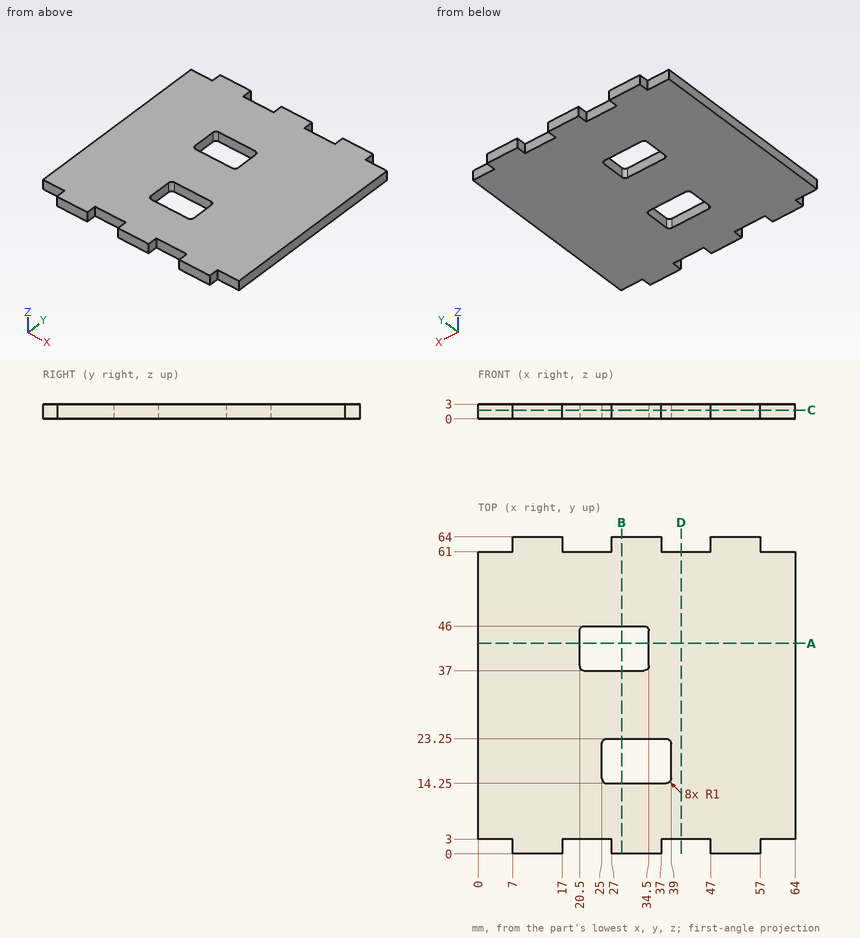
For this review, use the dimensioned drawing (mm, ordinates from the lowest corner) and the shaded views. Give positions to 0.01 mm unless a question says otherwise; leave off trailing zeros. Write each loop counter-clockwise with the first axis right and the second up, starting at its lowest first coordinate (ties: lowest second). Pieces come first, ordered by that corner, then holes. Notation, with made-up numbers: M -15,-13.75 L 21,-13.75 A18 ccw 21,-4.75 Z; hole C 2.25,44 d8. An arc over 180 degrees is marked long. Answer as a JSON object with one key per item and string values. Group by question number.
1) Clearance check with flat-ended pins moving along their axes: pin 1 Ø0.9 at (y, z) = (41, 1) entering from -X; pin 2 Ø1.5 at (y, z) = (63, 1) entering from +X; pin 3 Ø0.9 at (x, z) = (5, 2) entering from -Y. State where each tip first meets the part, or that it passes through.
2) We need section C-C (z = 1.75). Count the separate pieces of the cut face and the enclosed holes in it, and give its area (3 significant figures).
3) We need section A-A (y = 42.5). Give the boundary of the cut face in (x, z), and give its area (3 significant figures).
4) We need section D-D (x = 41). Give the boundary of the cut face in (y, z).
5) We need section B-B (x = 29). Give the boundary of the cut face in (y, z), and give its area (3 significant figures).
6) For line 1 along X through (y, z) = (42, 1.8); line 2 along Y through (x, z) = (24.5, 0.7); line 3 along Y through (x, z) = (25.5, 2.65), list the stretches that pass through material, from the lowest coordinate up.
Answer key:
{
 "1": {"pin 1": "stops at x = 0", "pin 2": "stops at x = 57", "pin 3": "stops at y = 3"},
 "2": {"separate pieces": "1", "enclosed holes": "2", "area": "3,640 mm²"},
 "3": {"outline": "M 0,0 L 20.5,0 L 20.5,3 L 0,3 Z; M 34.5,0 L 64,0 L 64,3 L 34.5,3 Z", "area": "150 mm²"},
 "4": {"outline": "M 3,0 L 61,0 L 61,3 L 3,3 Z"},
 "5": {"outline": "M 0,0 L 14.25,0 L 14.25,3 L 0,3 Z; M 23.25,0 L 37,0 L 37,3 L 23.25,3 Z; M 46,0 L 64,0 L 64,3 L 46,3 Z", "area": "138 mm²"},
 "6": {"line 1": "x = 0 to 20.5, 34.5 to 64", "line 2": "y = 3 to 37, 46 to 61", "line 3": "y = 3 to 14.38, 23.12 to 37, 46 to 61"}
}
